Geometry: final body of the model. Coordinates: model frame, mm. Coordinates: 2 decimals unless noted, no trailing zeros. Write each loop counter-clockwise with the first axis right and the second up, starting at its lowest first coordinate (ties: lowest second). Pieces come first, ordered by that corner, then holes.
Autodesk Inventor part; units mm, degrees
ref_plane "YZ Plane" through (0, 0, 0) normal (1, 0, 0) x (0, 1, 0)
ref_plane "XZ Plane" through (0, 0, 0) normal (0, 1, 0) x (-1, 0, 0)
ref_plane "XY Plane" through (0, 0, 0) normal (0, 0, 1) x (1, 0, 0)
sketch "Sketch1" plane through (0, 0, 0) normal (0, 0, 1) x (1, 0, 0)
  line L0 (0, 54.7703) -> (0, -37.28)
  line L1 (-15.2248, 0) -> (91.3486, 0)
  arc A0 (53.2038, -24.13) -> (42.5734, 40.005) centre (0, 0) ccw
  line L2 (42.5734, 40.005) -> (76.1238, 40.005)
  line L3 (76.1238, 40.005) -> (76.1238, -24.13)
  line L4 (53.2038, -24.13) -> (76.1238, -24.13)
  point P0 (68.1228, 16.51)
  point P1 (68.1228, 0)
  point P2 (68.1228, -16.51)
  dimension "d0" = 58.42
  dimension "d1" = 40.005
  dimension "d2" = 24.13
  dimension "d69" = 76.1238
  dimension "d133" = 8.001
  dimension "d134" = 16.51
  dimension "d135" = 16.51
  dimension "d145" = 33.5504
  dimension "d146" = 64.135
extrude "Extrusion1" add sketch "Sketch1" against normal blind 3.175
hole "Hole6" at (68.1228, 16.51, 0) at (68.1228, -16.51, 0) direction (0, 0, -1) diameter 2.4638 end through all
fillet "Fillet11" radius 3.81 1 edges at (53.2038, -24.13, -1.5875)
fillet "Fillet12" radius 6.35 2 edges at (76.1238, 40.005, -1.5875) (42.5734, 40.005, -1.5875)
properties part number "J005357" material "STEEL, LOW CARBON (1008/1018/1020)"
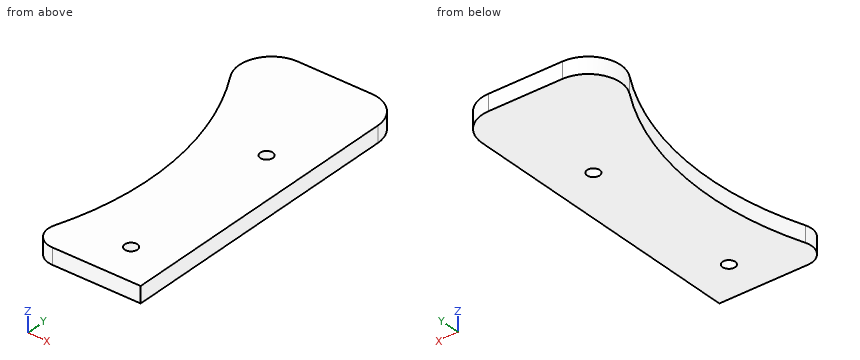
Item 1: Section D-D, the plane y = 26. Output: boundary loops of the cut face in (x, z) (3 decimals), plus the area to 3 significant figures.
Derived:
outline: (52.315, -3.175) - (76.124, -3.175) - (76.124, 0) - (52.315, 0) - close
area: 75.6 mm2
Item 2: Section B-B, the plane z = -1.25. Output: boundary loops of the cut face in (x, y) (3 decimals), plus the area to 3 significant figures.
Derived:
outline: (49.914, 30.355) arc R58.42 cw to (55.218, -19.076) arc R3.81 ccw to (58.819, -24.13) - (76.124, -24.13) - (76.124, 33.655) arc R6.35 ccw to (69.774, 40.005) - (55.34, 40.005) arc R6.35 ccw to start; hole circle Ø2.464 at (68.123, -16.51); hole circle Ø2.464 at (68.123, 16.51)
area: 1,320 mm2
Item 3: Section C-C, the plane y = -1. Output: boundary loops of the cut face in (x, z) (3 decimals), plus the area to 3 significant figures.
Derived:
outline: (58.411, -3.175) - (76.124, -3.175) - (76.124, 0) - (58.411, 0) - close
area: 56.2 mm2
Item 4: Material intervals for probe 1 along Y at (x, z) = (68, -0.7) (3 decimals); probe 2 along Y at (x, z) = (67.5, -0.3) (3 decimals); probe 3 along Y at (x, z) = (58.5, -0.7) (3 decimals), sorted ascending.
Derived:
probe 1: y = -24.13 to -17.736, -15.284 to 15.284, 17.736 to 40.005
probe 2: y = -24.13 to -17.573, -15.447 to 15.447, 17.573 to 40.005
probe 3: y = -24.117 to 40.005
Item 5: Section A-A, the plane y = 16.51. Output: boundary loops of the cut face in (x, z) (3 decimals).
Derived:
outline: (56.039, -3.175) - (66.891, -3.175) - (66.891, 0) - (56.039, 0) - close; (69.355, -3.175) - (76.124, -3.175) - (76.124, 0) - (69.355, 0) - close
